```python
from build123d import *

# Parameters (mm, degrees)
SKETCH1_W           = 61.321024484
SKETCH1_H           = 177.8
SKETCH1_R           = 8.89
SKETCH1_R_2         = 2.032
BOSS_EXTRUDE1_DEPTH = 19.05
BOSS_EXTRUDE2_DEPTH = 61.321024


with BuildPart() as part:
    # Sketch1 → Boss-Extrude1 (new body)
    with BuildSketch(Plane(origin=(0, 0, 0), x_dir=(0, 0, -1), z_dir=(1, 0, 0))):
        Rectangle(SKETCH1_W, SKETCH1_H)
        with Locations((0, 45.539487758)):
            Circle(SKETCH1_R, mode=Mode.SUBTRACT)
        with Locations((-17.960512242, 63.5)):
            Circle(SKETCH1_R_2, mode=Mode.SUBTRACT)
        with Locations((17.960512242, 27.578975516)):
            Circle(SKETCH1_R_2, mode=Mode.SUBTRACT)
    extrude(amount=BOSS_EXTRUDE1_DEPTH)

    # Sketch2 → Boss-Extrude2 (add)
    with BuildSketch(Plane.XY.offset(30.660512242)):
        Polygon((19.05, -88.9), (82.435420259, -88.9), (19.05, -83.82), align=None)
    extrude(amount=-BOSS_EXTRUDE2_DEPTH)


solid = part.part
```
Could you check a few things on this model? Use its own coordinates, in mm. A direction names the side the tool comes from. Coordinates: 2 decimals unless noted, no trailing zeros. Write each loop counter-clockwise with the first axis right and the second up, starting at its lowest first coordinate (ties: lowest second). Pieces come first, ordered by that corner, then holes. Notation, with made-up numbers: (5.5, 2.5) -> (34.5, 2.5) arc R20 ccw to (34.5, 36.5) -> close; hole circle Ø1 at (57, 43.25). An arc over 180 degrees is marked (long way). One line per question, with ' | ' between items. Start each with the question number.
1. If we section it at C-C (x = 72): Please give me the cut outline in (y, z).
2. If we section it at B-B (z = 0): Please give me the cut outline in (x, y).
3. If we section it at D-D (x = 40): Please give me the cut outline in (y, z), and give its area (3 significant figures).
4. Thinking about a two-plate mould opening in Z: for faces 3 (the face through (51.186, -86.396, 0.429)), 4 (the face through (10, -6, 30.661)), 5 (the face through (9.39, 36.86, 1.93)), which applies, pulls with the +Z half, pulls with the -Z half, needs draft (parallel to the pull), parting line crosses it, or undercut?
5. Please list where these lines run through material, in increasing order: line 1 along X through (y, z) = (-60, 6); line 2 along Z through (x, y) = (9, 63); line 3 along Y through (x, z) = (71, -17).
6. Will these pins go through, and if not, where does the flat tip stop? P1, Ø4, axis at y = 1, z = 16, coming from the -X side; P2, Ø20.5, axis at y = 45.54, z = 0, coming from the +X side; P3, Ø10, axis at x = 53.5, z = 7, coming from the +Y side; P4, Ø4, axis at x = 41, z = -15.5, coming from the +Y side.
7. For faces 1 (the face through (19.05, 1, 0)), 2 (the face through (41, -88.9, 0)), which set-ups out of +Z, -Z, +X, -X, +Y, -Y let a thin tool reach every point of the face, with its end or its side?
8. If we section it at A-A (y = 63.5): Please give me the cut outline in (x, z).
Return value:
1) outline: (-88.9, -30.66) -> (-88.06, -30.66) -> (-88.06, 30.66) -> (-88.9, 30.66) -> close
2) outline: (0, -88.9) -> (82.44, -88.9) -> (19.05, -83.82) -> (19.05, 36.65) -> (0, 36.65) -> close; (0, 54.43) -> (19.05, 54.43) -> (19.05, 88.9) -> (0, 88.9) -> close
3) outline: (-88.9, -30.66) -> (-85.5, -30.66) -> (-85.5, 30.66) -> (-88.9, 30.66) -> close | area: 209 mm²
4) face 3: needs draft | face 4: pulls with the +Z half | face 5: undercut
5) line 1: x = 0 to 19.05 | line 2: z = -30.66 to 15.99, 19.93 to 30.66 | line 3: y = -88.9 to -87.98
6) P1: stops at x = 0 | P2: stops at x = 19.05 | P3: stops at y = -86.18 | P4: stops at y = -85.42
7) face 1: +Z, -Z, +X, +Y | face 2: +Z, -Z, +X, -X, -Y
8) outline: (0, -30.66) -> (19.05, -30.66) -> (19.05, 15.93) -> (0, 15.93) -> close; (0, 19.99) -> (19.05, 19.99) -> (19.05, 30.66) -> (0, 30.66) -> close
